The drawing under review shows one solid part. Ordinate dimensions are in mm from its lowest x, y, z. A direction names the side the tool comes from. Coordinates: 2 decimals unless noted, no trailing zeros. Loops run counter-clockwise (first coordinate to the right, second up) from the corner with the lowest first, then second, coordinate; pieces in that order, holes last. Notation, with made-up numbers: M 35.5,-35 L 78.5,-35 A22 cw 78.5,-11 Z; hole C 5,24 d11. An arc over 180 degrees is marked long. Return JSON: item names as keys, results as strings.
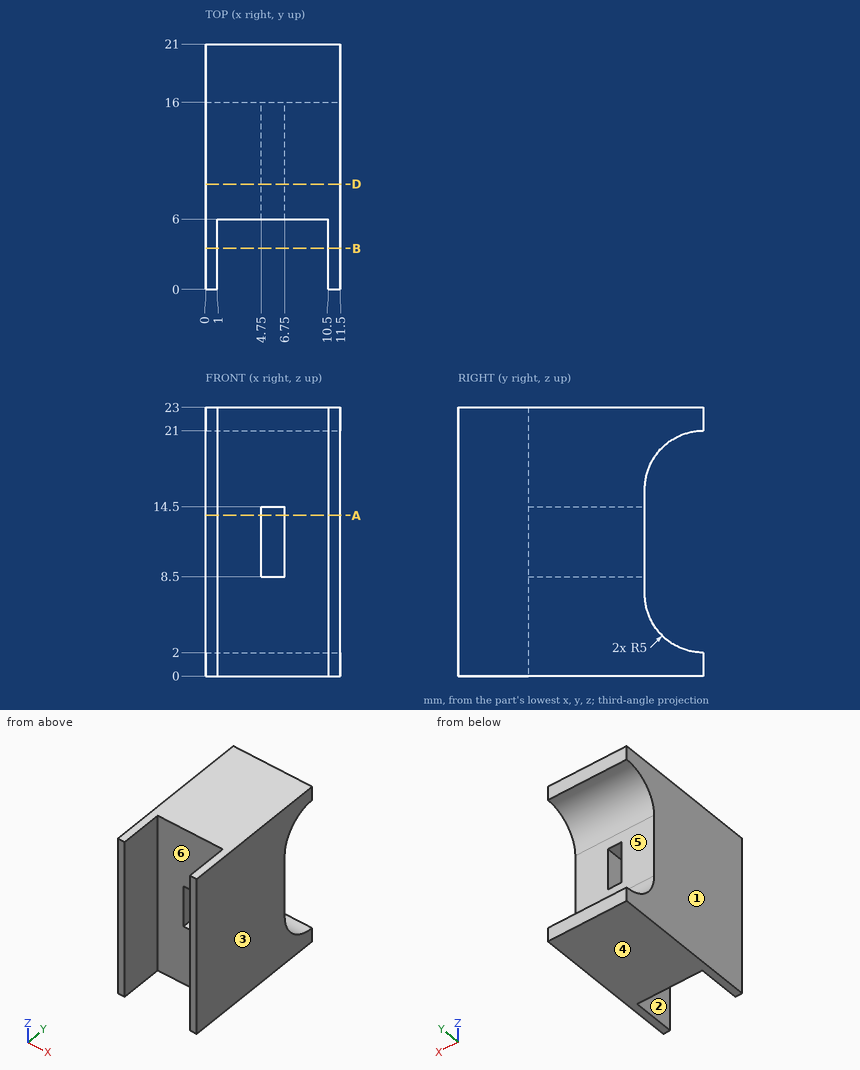
1. The part is to be moulded in two halves that separate along X. For the marked faces 1, 2 and 3, say which applies: released by +X, released by -X, zero draft, split by the parting line, or undercut.
Check values:
{"face 1": "released by -X", "face 2": "undercut", "face 3": "released by +X"}
2. Add section D-D on y = 9. Give the boundary of the cut face in (x, z), plus the area to 4 significant figures.
Check values:
{"outline": "M 0,0 L 11.5,0 L 11.5,23 L 0,23 Z; hole M 4.75,8.5 L 6.75,8.5 L 6.75,14.5 L 4.75,14.5 Z", "area": "252.5 mm²"}
3. Add section B-B on y = 3.5. Give the boundary of the cut face in (x, z), plus the area to 3 significant figures.
Check values:
{"outline": "M 0,0 L 1,0 L 1,23 L 0,23 Z; M 10.5,0 L 11.5,0 L 11.5,23 L 10.5,23 Z", "area": "46.0 mm²"}
4. Add section A-A on z = 13.75. Give the boundary of the cut face in (x, y).
Check values:
{"outline": "M 0,0 L 1,0 L 1,6 L 4.75,6 L 4.75,16 L 0,16 Z; M 6.75,6 L 10.5,6 L 10.5,0 L 11.5,0 L 11.5,16 L 6.75,16 Z"}
5. Insertion check: pin 1 Ø3 at (x, z) = (6.5, 7.5) entering from -Y. The pin has a flat end and moves straight along its axis. Give the tip position at first contact, or say it passes through.
Check values:
{"pin 1": "y = 6"}
6. To check wall thickness, follow line 1 (Y direction, x = 6.75, z = 7.75); line 2 (X direction, y = 3.5, z = 5); line 3 (Y direction, x = 2, z = 18.75). State the ranges of each line that lie inside material, in increasing order.
Check values:
{"line 1": "6 to 16", "line 2": "0 to 1, 10.5 to 11.5", "line 3": "6 to 16.82"}
7. Machinability: for the marked faces 4, 5 and 6, which of the approach directions +Z, -Z, +X, -X, +Y, -Y give a long, thin tool a straight path to every point of the face, cutting with its end or side? Answer none if there is none.
Check values:
{"face 4": "-Z, +X, -X, +Y, -Y", "face 5": "+X, -X, +Y", "face 6": "+Z, -Z, -Y"}
